Autodesk Inventor part; units mm, degrees
ref_plane "YZ Plane" through (0, 0, 0) normal (1, 0, 0) x (0, 1, 0)
ref_plane "XZ Plane" through (0, 0, 0) normal (0, 1, 0) x (-1, 0, 0)
ref_plane "XY Plane" through (0, 0, 0) normal (0, 0, 1) x (1, 0, 0)
sketch "Sketch1" plane through (0, 0, 0) normal (0, 0, 1) x (1, 0, 0)
  line L0 (51.2872, 31.5555) -> (51.2872, -28.4445)
  line L1 (16.2872, 31.5555) -> (16.2872, -28.4445)
  arc A0 (16.2872, -28.4445) -> (-8.7128, -71.7458) centre (78.6621, -93.3242) ccw
  line L2 (16.2872, -28.4445) -> (-8.7128, -71.7458) construction
  line L3 (16.2872, -28.4445) -> (66.2872, -28.4445) construction
  line L4 (-8.7128, -71.7458) -> (-8.7128, -121.7458)
  arc A1 (76.1491, -71.1938) -> (51.2872, -28.4445) centre (-11.0876, -93.3242) ccw
  line L5 (76.1491, -71.1938) -> (76.1491, -121.1332)
  line L6 (26.2872, -121.7458) -> (26.2872, -76.5352)
  arc A2 (33.7872, -61.5241) -> (26.2872, -76.5352) centre (78.6621, -93.3242) ccw
  arc A3 (41.1491, -76.1101) -> (33.7872, -61.5241) centre (-11.0876, -93.3242) ccw
  line L7 (41.1491, -76.1101) -> (41.1491, -121.1332)
  line L8 (-18.7128, -121.1332) -> (-18.7128, -70.5617)
  arc A4 (6.2872, -24.3178) -> (-18.7128, -70.5617) centre (78.6621, -93.3242) ccw
  line L9 (6.2872, -24.3178) -> (6.2872, 37.168)
  line L10 (6.2872, 37.168) -> (61.2872, 37.168)
  line L11 (61.2872, 37.168) -> (61.2872, -24.3178)
  arc A5 (86.1491, -69.9786) -> (61.2872, -24.3178) centre (-11.0876, -93.3242) ccw
  line L12 (86.1491, -69.9786) -> (86.1491, -121.1332)
  line L13 (-18.7128, -121.1332) -> (86.1491, -121.1332)
  line L14 (16.2872, 31.5555) -> (16.2872, 37.168)
  line L15 (51.2872, 31.5555) -> (51.2872, 37.168)
  line L16 (36.1491, -121.1332) -> (36.1491, -85.5895)
  line L17 (31.2872, -85.5895) -> (31.2872, -121.7458)
  line L18 (26.2872, -85.5895) -> (31.2872, -85.5895)
  line L19 (36.1491, -85.5895) -> (41.1491, -85.5895)
  line L20 (50.9283, 31.5555) -> (51.2872, 31.5555)
  line L21 (16.2872, 2.168) -> (16.2872, 22.168)
  line L22 (51.2872, 2.168) -> (51.2872, 22.168)
  line L23 (76.1491, -101.1332) -> (76.1491, -81.1332)
  line L24 (-8.7128, -81.1332) -> (-8.7128, -101.1332)
  line L25 (78.6491, -80.1332) -> (83.6491, -80.1332)
  line L26 (83.6491, -80.1332) -> (83.6491, -101.1332)
  line L27 (83.6491, -101.1332) -> (78.6491, -101.1332)
  line L28 (78.6491, -101.1332) -> (78.6491, -80.1332)
  line L29 (-16.1906, -80.1332) -> (-11.1906, -80.1332)
  line L30 (-11.1906, -80.1332) -> (-11.1906, -101.1332)
  line L31 (-11.1906, -101.1332) -> (-16.1906, -101.1332)
  line L32 (-16.1906, -101.1332) -> (-16.1906, -80.1332)
  line L33 (53.7872, 22.168) -> (58.7872, 22.168)
  line L34 (58.7872, 22.168) -> (58.7872, 1.168)
  line L35 (58.7872, 1.168) -> (53.7872, 1.168)
  line L36 (53.7872, 1.168) -> (53.7872, 22.168)
  line L37 (8.7872, 22.168) -> (13.7872, 22.168)
  line L38 (13.7872, 22.168) -> (13.7872, 1.168)
  line L39 (13.7872, 1.168) -> (8.7872, 1.168)
  line L40 (8.7872, 1.168) -> (8.7872, 22.168)
  point P0 (0, 0)
  point P1 (-8.7128, -121.1332)
  point P2 (26.2872, -121.1332)
  point P3 (36.2872, -121.7458)
  point P4 (71.2872, -121.7458)
  point P5 (31.2872, -121.1332)
  point P6 (31.2872, -121.7458)
  dimension "d0" = 35
  dimension "d1" = 60
  dimension "d2" = 50
  dimension "d3" = 120
  dimension "d4" = 90
  dimension "d5" = 50
  dimension "d6" = 35
  dimension "d7" = 10
  dimension "d12" = 5
  dimension "d16" = 10
  dimension "d22" = 158.3013
  dimension "d29" = 0
  dimension "d30" = 5
  dimension "d31" = 21
  dimension "d32" = 5
  dimension "d33" = 21
  dimension "d34" = 5
  dimension "d35" = 21
  dimension "d36" = 5
  dimension "d37" = 21
  dimension "d38" = 2.5
  dimension "d39" = 15
  dimension "d40" = 2.5
  dimension "d41" = 15
  dimension "d42" = 20
  dimension "d43" = 20
extrude "Extrusion1" add sketch "Sketch1" along normal blind 5 contours L15 L10 L11 A5 L12 L13 L5 A1 L0 | L0 A1 L5 L13 L7 A3 A2 L6 L4 A0 L1 L14 L10 L15 | L14 L1 A0 L4 L13 L8 A4 L9 L10
equation "\"d16\" = d7"
properties part number "newmiddle"
Check sheet for the modelled part. Datum: model origin and axes. Units: mm. A direction names the side the tool comes from. Give positions to 0.01 mm unless a question says otherwise; leave off trailing zeros. Write each loop counter-clockwise with the first axis right and the second up, starting at its lowest first coordinate (ties: lowest second). Pieces come first, ordered by that corner, then holes. Notation, with made-up numbers: (-22, 15.25) -> (14, 15.25) arc R12 cw to (14, 37.25) -> close; hole circle Ø8 at (43, 82.25). An arc over 180 degrees is marked (long way). Write item = value, one per line.
Item 1: Sectioned sample at C-C on z = 3.1. Count the separate pieces of the cut face and the enclosed holes in it, and give its area (3 significant figures).
Output:
separate_pieces = 1
enclosed_holes = 4
area = 11,400 mm^2
Item 2: Sectioned sample at A-A on y = 15. Record the boundary of the cut face in (x, z), and give its area (3 significant figures).
Output:
outline = (6.29, 0) -> (8.79, 0) -> (8.79, 5) -> (6.29, 5) -> close; (13.79, 0) -> (53.79, 0) -> (53.79, 5) -> (13.79, 5) -> close; (58.79, 0) -> (61.29, 0) -> (61.29, 5) -> (58.79, 5) -> close
area = 225 mm^2
Item 3: Release check for a two-part mould opening along Y. For faces 6 (the flat face through (56, 1.168, 2)), 7 (the flat face through (3, -121.133, 2)), 8 (the flat face through (86.149, -95, 2)) record: +Y half, -Y half, draft (parallel to the pull), parting line (faces both ways), or undercut.
Output:
face_6 = undercut
face_7 = -Y half
face_8 = draft
Item 4: Gauge pin test, flat ends, axial feed: pin 1 (1 mm diameter, centred on x = 32, z = 3.5, fed in from -Y); pin 2 (1 mm diameter, centred on x = 5, z = 3.5, fed in from +Y); pin 3 (2.5 mm diameter, centred on y = 9, z = 1.5, fed in from -X). Record the tip position at first contact, or that the pin passes through.
Output:
pin_1 = -65.03
pin_2 = -25.15
pin_3 = 6.29
Item 5: Sectioned sample at B-B on y = -104.5. Record the boundary of the cut face in (x, z), and give its area (3 significant figures).
Output:
outline = (-18.71, 0) -> (26.29, 0) -> (26.29, 5) -> (-18.71, 5) -> close; (41.15, 0) -> (86.15, 0) -> (86.15, 5) -> (41.15, 5) -> close
area = 450 mm^2
Item 6: Sectioned sample at D-D on y = -20. Record the boundary of the cut face in (x, z), and give its area (3 significant figures).
Output:
outline = (6.29, 0) -> (61.29, 0) -> (61.29, 5) -> (6.29, 5) -> close
area = 275 mm^2
Item 7: Tool access check on faces 1 (the flat face through (33, 37.168, 2)), 2 (the flat face through (41.149, -98, 2)), 3 (the flat face through (6.287, 6, 2)), 4 (the flat face through (11, 22.168, 2)), 5 (the flat face through (61.287, 7, 2)). Record the directions out of +Z, -Z, +X, -X, +Y, -Y that give a thin tool (end or side, any length) a straight path to the whole face; none if there is none.
Output:
face_1 = +Z, -Z, +X, -X, +Y
face_2 = +Z, -Z, -Y
face_3 = +Z, -Z, -X, +Y
face_4 = +Z, -Z
face_5 = +Z, -Z, +X, +Y
Item 8: Scan lines: probe 1 along X at (y, z) = (5, 2.6); probe 2 along X at (y, z) = (-81, 1.8); probe 3 along X at (y, z) = (-17, 1.4). Record each from-to range of solid material in increasing order. Write a range as from..to.
Output:
probe_1 = 6.29..8.79, 13.79..53.79, 58.79..61.29
probe_2 = -18.71..-16.19, -11.19..26.29, 41.15..78.65, 83.65..86.15
probe_3 = 6.29..61.29
